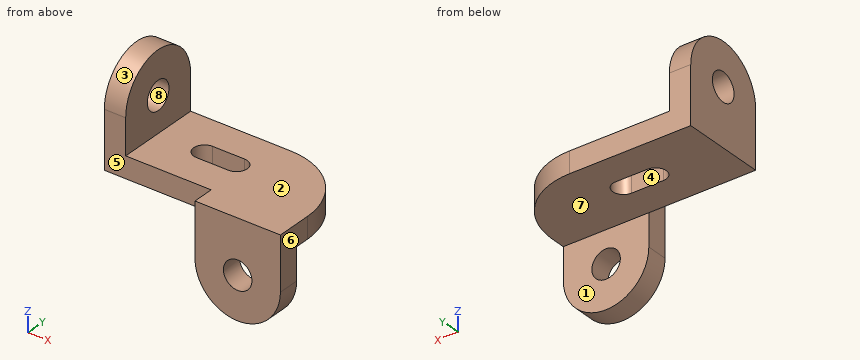
```python
from build123d import *

# Parameters (mm, degrees)
F0_W      = 121.92
F0_H      = 60.96
F0_W_2    = 15.24
F1_DEPTH  = 15.24
F2_DEPTH  = 25.4
F4_DEPTH  = 15.24
F5_DEPTH  = 15.241
F6_W      = 60.96
F6_H      = 15.24
F7_DEPTH  = 15.24
F8_R      = 50.8
F9_W      = 22.86
F9_H      = 15.24
F10_DEPTH = 68.581


with BuildPart() as f1:
    # F0 (on Top) → F1 (new body)
    with BuildSketch(Plane.XY):
        with Locations((7.62, 0)):
            Rectangle(F0_W, F0_H)
        with Locations((-60.96, 0)):
            Rectangle(F0_W_2, F0_H)
    extrude(amount=-F1_DEPTH)

    # F0 (on Top) → F2 (join)
    with BuildSketch(Plane.XY):
        with Locations((-60.96, 0)):
            Rectangle(F0_W_2, F0_H)
    extrude(amount=F2_DEPTH)

    # F3 (on face) → F4 (join)
    with BuildSketch(Plane.YZ.offset(-53.34)):
        with BuildLine():
            Line((10.16, 25.4), (30.48, 25.4))
            ThreePointArc((30.48, 25.4), (0, 55.88), (-30.48, 25.4))
            Line((-30.48, 25.4), (-10.16, 25.4))
            ThreePointArc((-10.16, 25.4), (0, 35.56), (10.16, 25.4))
        make_face()
    extrude(amount=-F4_DEPTH)

    # F3 (on face) → F5 (cut, through all)
    with BuildSketch(Plane.YZ.offset(-53.34)):
        with BuildLine():
            ThreePointArc((-10.16, 25.4), (0, 15.24), (10.16, 25.4))
            Line((10.16, 25.4), (-10.16, 25.4))
        make_face()
        with BuildLine():
            Line((-10.16, 25.4), (10.16, 25.4))
            ThreePointArc((10.16, 25.4), (0, 35.56), (-10.16, 25.4))
        make_face()
    extrude(amount=-F5_DEPTH, mode=Mode.SUBTRACT)

    # F6 (on face) → F7 (join)
    with BuildSketch(Plane.XZ.offset(30.48)):
        with Locations((38.1, -7.62)):
            Rectangle(F6_W, F6_H)
        with BuildLine():
            Line((68.58, -38.1), (68.58, -15.24))
            Line((68.58, -15.24), (7.62, -15.24))
            Line((7.62, -15.24), (7.62, -38.1))
            Line((7.62, -38.1), (27.94, -38.1))
            ThreePointArc((27.94, -38.1), (38.1, -27.94), (48.26, -38.1))
            Line((48.26, -38.1), (68.58, -38.1))
        make_face()
        with BuildLine():
            ThreePointArc((7.62, -38.1), (38.1, -68.58), (68.58, -38.1))
            Line((68.58, -38.1), (48.26, -38.1))
            ThreePointArc((48.26, -38.1), (38.1, -48.26), (27.94, -38.1))
            Line((27.94, -38.1), (7.62, -38.1))
        make_face()
    extrude(amount=F7_DEPTH)

    # F8
    f8_edges = [f1.edges().sort_by_distance(p)[0] for p in [
        (68.58, 30.48, -7.62),
    ]]
    fillet(f8_edges, radius=F8_R)

    # F9 (on face) → F10 (cut, through all)
    with BuildSketch(Plane.XY):
        with Locations((-8.89, 0)):
            Rectangle(F9_W, F9_H)
        with BuildLine():
            Line((2.54, 7.62), (2.54, -7.62))
            ThreePointArc((2.54, -7.62), (10.16, 0), (2.54, 7.62))
        make_face()
        with BuildLine():
            ThreePointArc((-20.32, 7.62), (-27.94, 0), (-20.32, -7.62))
            Line((-20.32, -7.62), (-20.32, 7.62))
        make_face()
    extrude(amount=-F10_DEPTH, mode=Mode.SUBTRACT)


solid = f1.part
```
The model under review builds one solid part; all positions refer to its coordinate system, in mm. Face numbers are marked on the shaded views. A direction names the side the tool comes from. Coordinates: 2 decimals unless noted, no trailing zeros. Order: outer loops, then holes, each group sorted by start corner. A loop starts at its lowest first (then second) coordinate and runs counter-clockwise, first axis right, second up. Notation, with made-up numbers: (36, 1) -> (42, 1) arc R24 cw to (42, 37) -> close; hole circle Ø3 at (-1, -14). An arc over 180 degrees is marked (long way). Answer in a Markdown table with one row per item. Add a question column.
Item 1: We need section A-A on x = -6.5. Write out the cut boundary in (y, z), plus the area to 3 significant figures.
Item 2: Mouldability with a two-part tool opening along Z and no side actions: class the marked faces 6, 7 and 8 as +Z half, -Z half, draft (parallel to the pull), parting line (faces both ways), or undercut.
Item 3: We need section C-C on y = 0. Write out the cut boundary in (x, z).
Item 4: To check wall thickness, follow probe 1 along Y at (x, z) = (-61, 25.4); probe 2 along X at (y, z) = (-37.5, -38.1); probe 3 along Z at (x, y) = (-61, 0). State the ranges of each line that lie inside material, in increasing order.
Item 5: Machinability: for the marked faces 1, 2, 3, 4 and 5, which of the approach directions +Z, -Z, +X, -X, +Y, -Y give a long, thin tool a straight path to every point of the face, cutting with its end or side? Answer none if there is none.
Item 6: We need section D-D on z = -45. Write out the cut boundary in (x, y), plus the area to 3 significant figures.
Item 7: Clearance check with flat-ended pins moving along their axes: pin 1 (18.5 mm diameter, centred on y = 0, z = 25.4, fed in from +X); pin 2 (8 mm diameter, centred on x = 48.5, z = -41, fed in from +Y); pin 3 (18.5 mm diameter, centred on x = -13.5, y = -9, fed in from -Z); pin 4 (7.5 mm diameter, centred on x = -3, z = -11.5, fed in from -Y). State where each tip first meets the part, or that it passes through.
Item 8: We need section B-B on z = -5. Write out the cut boundary in (x, y).
Final values:
| question | item | result |
|---|---|---|
| 1 | outline | (-30.48, -15.24) -> (-7.62, -15.24) -> (-7.62, 0) -> (-30.48, 0) -> close; (7.62, -15.24) -> (30.48, -15.24) -> (30.48, 0) -> (7.62, 0) -> close |
| 1 | area | 697 mm2 |
| 2 | face 6 | draft |
| 2 | face 7 | -Z half |
| 2 | face 8 | undercut |
| 3 | outline | (-68.58, -15.24) -> (-27.94, -15.24) -> (-27.94, 0) -> (-53.34, 0) -> (-53.34, 15.24) -> (-68.58, 15.24) -> close; (-68.58, 35.56) -> (-53.34, 35.56) -> (-53.34, 55.88) -> (-68.58, 55.88) -> close; (10.16, -15.24) -> (64.34, -15.24) -> (64.34, 0) -> (10.16, 0) -> close |
| 4 | probe 1 | y = -30.48 to -10.16, 10.16 to 30.48 |
| 4 | probe 2 | x = 7.62 to 27.94, 48.26 to 68.58 |
| 4 | probe 3 | z = -15.24 to 15.24, 35.56 to 55.88 |
| 5 | face 1 | -Z, +X, -X, +Y |
| 5 | face 2 | +Z, +X, +Y, -Y |
| 5 | face 3 | +Z, +X, -X |
| 5 | face 4 | +Z, -Z |
| 5 | face 5 | +Z, -Z, -X, -Y |
| 6 | outline | (8.41, -45.72) -> (30.64, -45.72) -> (30.64, -30.48) -> (8.41, -30.48) -> close; (45.56, -45.72) -> (67.79, -45.72) -> (67.79, -30.48) -> (45.56, -30.48) -> close |
| 6 | area | 678 mm2 |
| 7 | pin 1 | passes through |
| 7 | pin 2 | stops at y = -30.48 |
| 7 | pin 3 | stops at z = -15.24 |
| 7 | pin 4 | stops at y = -30.48 |
| 8 | outline | (-68.58, -30.48) -> (7.62, -30.48) -> (7.62, -45.72) -> (68.58, -45.72) -> (68.58, -20.32) arc R50.8 ccw to (17.78, 30.48) -> (-68.58, 30.48) -> close; hole (-20.32, -7.62) -> (2.54, -7.62) arc R7.62 ccw to (2.54, 7.62) -> (-20.32, 7.62) arc R7.62 ccw to start |
